Input: part model. Units: mm. Frame: model coordinates. A direction names the side the tool comes from. Coordinates: 2 decimals unless noted, no trailing zeros. Order: outer loops, then holes, each group sorted by start corner. A loop starts at its lowest first (then second) coordinate and runs counter-clockwise, first axis right, second up. Notation, with made-up numbers: (57, 74) - (81, 74) arc R12 cw to (81, 96) - close; hole circle Ø6 at (-23, 10.25). An arc over 180 degrees is marked (long way). One line per question, with ' | ' between items.
from build123d import *

# Parameters (mm, degrees)
SKETCH_1_R      = 0.7835
EXTRUDE_1_DEPTH = 10
EXTRUDE_2_DEPTH = 10


with BuildPart() as part:
    # 草图1 → 凸台-拉伸1 (new body)
    with BuildSketch(Plane(origin=(0, 0, 0), x_dir=(0, 0, -1), z_dir=(1, 0, 0))):
        with BuildLine():
            Line((0, 0), (40, 0))
            Line((40, 0), (40, 240))
            ThreePointArc((40, 240), (37.071067812, 247.071067812), (30, 250))
            Line((30, 250), (10, 250))
            ThreePointArc((10, 250), (2.928932188, 247.071067812), (0, 240))
            Line((0, 240), (0, 0))
        make_face()
        with Locations((10, 235)):
            Circle(SKETCH_1_R, mode=Mode.SUBTRACT)
        with Locations((20, 235)):
            Circle(SKETCH_1_R, mode=Mode.SUBTRACT)
        with Locations((30, 235)):
            Circle(SKETCH_1_R, mode=Mode.SUBTRACT)
        with Locations((10, 194.5)):
            Circle(SKETCH_1_R, mode=Mode.SUBTRACT)
        with Locations((20, 194.5)):
            Circle(SKETCH_1_R, mode=Mode.SUBTRACT)
        with Locations((30, 194.5)):
            Circle(SKETCH_1_R, mode=Mode.SUBTRACT)
        with Locations((10, 154)):
            Circle(SKETCH_1_R, mode=Mode.SUBTRACT)
        with Locations((20, 154)):
            Circle(SKETCH_1_R, mode=Mode.SUBTRACT)
        with Locations((30, 154)):
            Circle(SKETCH_1_R, mode=Mode.SUBTRACT)
        with Locations((10, 113.5)):
            Circle(SKETCH_1_R, mode=Mode.SUBTRACT)
        with Locations((20, 113.5)):
            Circle(SKETCH_1_R, mode=Mode.SUBTRACT)
        with Locations((30, 113.5)):
            Circle(SKETCH_1_R, mode=Mode.SUBTRACT)
    extrude(amount=EXTRUDE_1_DEPTH)

    # 草图2 → 凸台-拉伸2 (add)
    with BuildSketch(Plane.XZ):
        with BuildLine():
            Line((-20, 30), (30, 30))
            ThreePointArc((30, 30), (37.071067812, 27.071067812), (40, 20))
            Line((40, 20), (40, -60))
            ThreePointArc((40, -60), (37.071067812, -67.071067812), (30, -70))
            Line((30, -70), (-20, -70))
            ThreePointArc((-20, -70), (-27.071067812, -67.071067812), (-30, -60))
            Line((-30, -60), (-30, 20))
            ThreePointArc((-30, 20), (-27.071067812, 27.071067812), (-20, 30))
        make_face()
    extrude(amount=EXTRUDE_2_DEPTH)


solid = part.part
Item 1: Contact query for flat-ended pins moving along their axis: P1, Ø0.9, axis at y = 235, z = -30, coming from the +X side; P2, Ø2.5, axis at y = 113.5, z = -30, coming from the -X side; P3, Ø5, axis at x = 5.5, y = 104, coming from the +Z side; P4, Ø10, axis at x = 8.5, z = -53.5, coming from the +Y side. Output: stop coordinate, or through.
Data:
P1: through | P2: x = 0 | P3: z = 0 | P4: y = 0
Item 2: Section B-B on x = -14.5. Return the cut outline in (y, z), and give its area (3 significant figures).
Data:
outline: (-10, -70) - (0, -70) - (0, 30) - (-10, 30) - close | area: 1,000 mm^2
Item 3: Section C-C on y = 98. Return the cut outline in (x, z), and give its area (3 significant figures).
Data:
outline: (0, -40) - (10, -40) - (10, 0) - (0, 0) - close | area: 400 mm^2
Item 4: Ray query, line 1 (Y direction, x = 5, z = -10); line 2 (Z direction, x = 3.75, y = 113.5); line 3 (Y direction, x = 31.5, z = -56.5). Return the intervals inside material, ascending.
Data:
line 1: -10 to 112.72, 114.28 to 153.22, 154.78 to 193.72, 195.28 to 234.22, 235.78 to 250 | line 2: -40 to -30.78, -29.22 to -20.78, -19.22 to -10.78, -9.22 to 0 | line 3: -10 to 0
Item 5: Section A-A on z = -5. Return the cut outline in (x, y).
Data:
outline: (-30, -10) - (40, -10) - (40, 0) - (10, 0) - (10, 248.66) - (0, 248.66) - (0, 0) - (-30, 0) - close
Item 6: Access query for faces 1 (the face through (5, 118, -40)), 2 (the face through (5, 122, 0)), 3 (the face through (0, 127, -20)), 4 (the face through (10, 127, -20)). Directions: +Z, -Z, +X, -X, +Y, -Y. A direction counts if a zero-diameter tool reaches every point of the face in a straight line with its end or side. Return the directions, or none.
Data:
face 1: -Z, +X, -X, +Y | face 2: +Z, +X, -X, +Y | face 3: +Z, -Z, -X, +Y | face 4: +Z, -Z, +X, +Y
